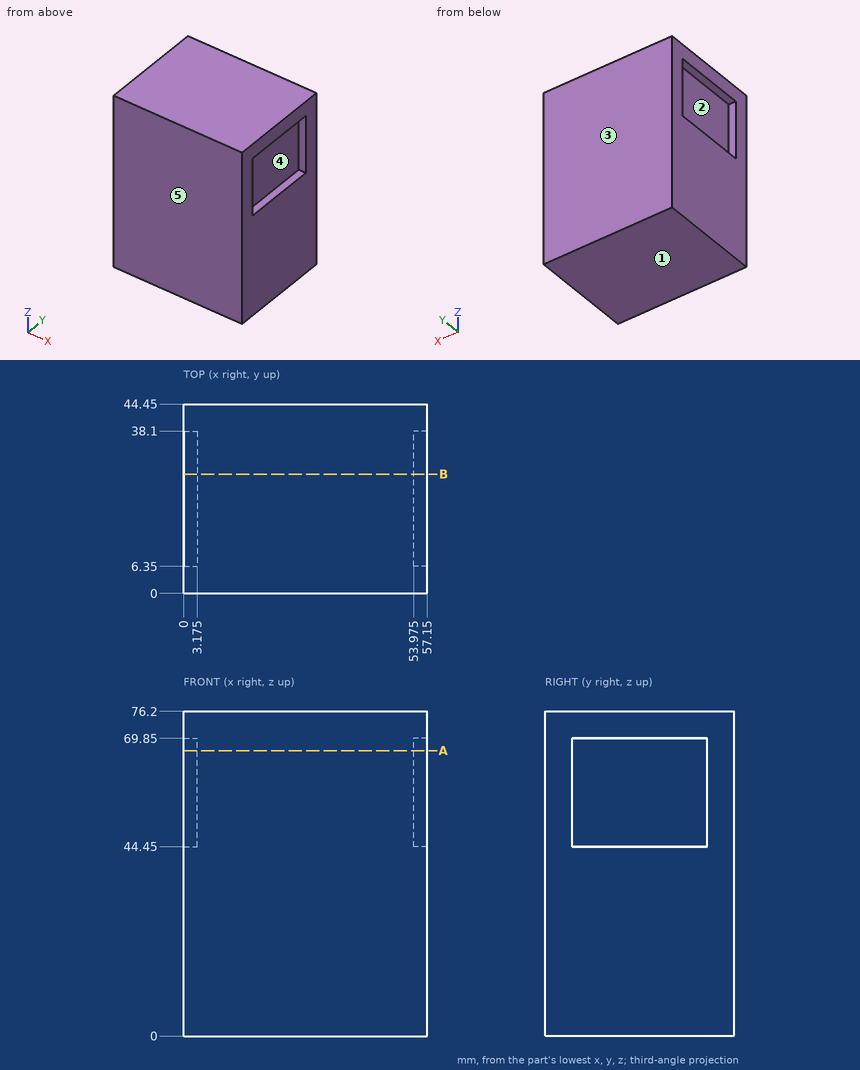
Can you work these out from the drawing? Everything is in mm from the part's minimum corner. A direction names the side the tool comes from. Coordinates: 2 decimals unless noted, no trailing zeros. Write each loop counter-clockwise with the first axis right and the second up, starting at its lowest first coordinate (ties: lowest second). Pieces come first, ordered by that corner, then holes. Notation, with made-up numbers: (-12, 58.25) - (34, 58.25) arc R20 cw to (34, 72.25) - close; hole circle Ø8 at (52.25, -31.5). An arc over 180 degrees is marked (long way). One line per item, written item: value.
1) Suppose I cut it at A-A on z = 67. Write out the boundary of the cut face in (x, y) (3 decimals), and give its area (3 significant figures).
Model answer:
outline: (0, 0) - (57.15, 0) - (57.15, 6.35) - (53.975, 6.35) - (53.975, 38.1) - (57.15, 38.1) - (57.15, 44.45) - (0, 44.45) - (0, 38.1) - (3.175, 38.1) - (3.175, 6.35) - (0, 6.35) - close
area: 2,340 mm²
2) Suppose I cut it at B-B on y = 28. Write out the boundary of the cut face in (x, z) (3 decimals), and give its area (3 significant figures).
Model answer:
outline: (0, 0) - (57.15, 0) - (57.15, 44.45) - (53.975, 44.45) - (53.975, 69.85) - (57.15, 69.85) - (57.15, 76.2) - (0, 76.2) - (0, 69.85) - (3.175, 69.85) - (3.175, 44.45) - (0, 44.45) - close
area: 4,190 mm²
3) I need wall thicknesses on line 1 along Y through (x, z) = (2, 52.5); line 2 along X through (y, z) = (18, 47) (3 decimals). Which ranges of each line are inside material? Lowest first, please.
Model answer:
line 1: y = 0 to 6.35, 38.1 to 44.45
line 2: x = 3.175 to 53.975
4) We'd pull the mould along Y, two halves only. Please class the marked faces 1, 2 and 3: pulls with the +Y half, pulls with the -Y half, needs draft (parallel to the pull), parting line crosses it, or undercut.
Model answer:
face 1: needs draft
face 2: undercut
face 3: pulls with the +Y half
5) I'm going to push flat-ended pins straight in: P1, Ø7.5, axis at y = 15.5, z = 56.5, coming from the +X side (3 decimals); P2, Ø12.5, axis at y = 18.5, z = 53.5, coming from the -X side (3 decimals). Where does each tip first touch, or does it pass through?
Model answer:
P1: stops at x = 53.975
P2: stops at x = 3.175
6) On a 3-axis mill with a long thin cutter (end or side, diameter ignored), from which of +Z, -Z, +X, -X, +Y, -Y can I reach the whole of each face in a straight line? I mean the marked faces 4 and 5. Say none if no direction works.
Model answer:
face 4: +X
face 5: +Z, -Z, +X, -X, -Y
